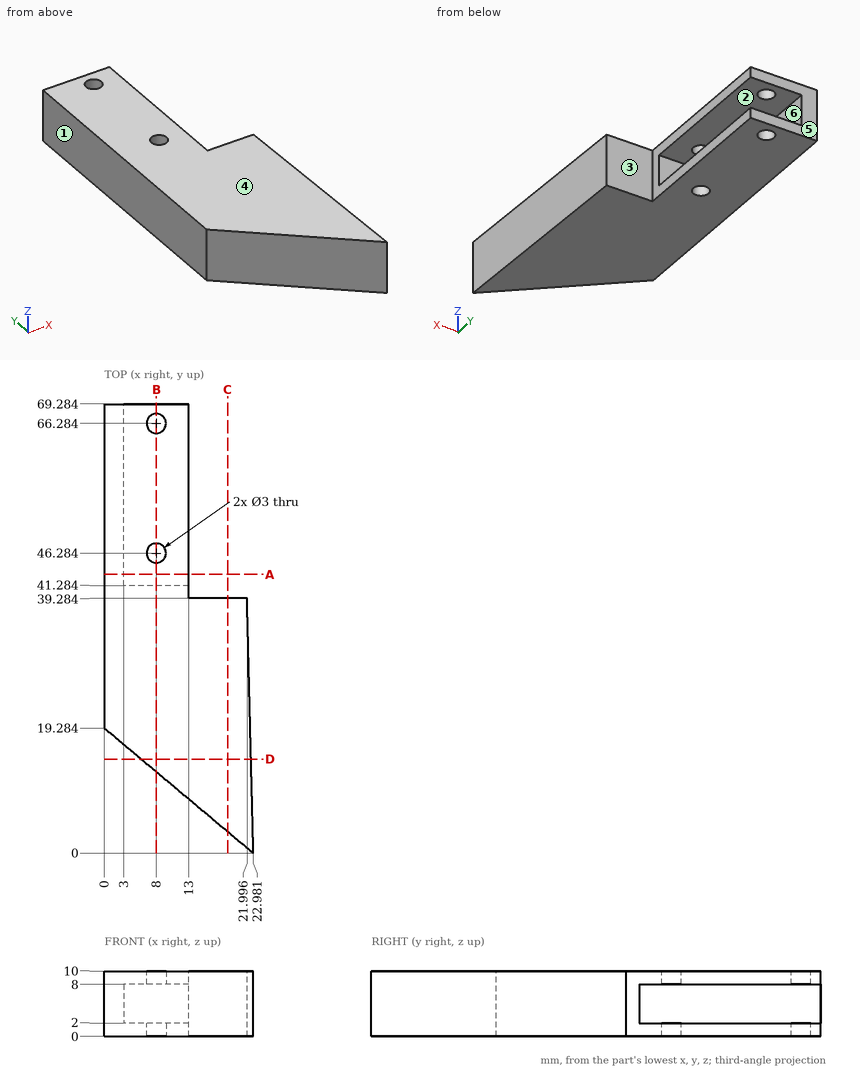
Verification items for this drawing (mm, ordinates from the low corner). A direction names the side the tool comes from. Give positions to 0.01 mm unless a question says otherwise; leave off trailing zeros. Loops run counter-clockwise (first coordinate to the right, second up) from the corner with the lowest first, then second, coordinate; pieces in that order, holes last. Notation, with made-up numbers: M 55,31.25 L 77,31.25 A25 cw 77,48.25 Z; hole C -7.75,48.25 d11. An arc over 180 degrees is marked long. Answer as CSV lines item,"result".
Item 1: Access from +Z, -Z, +X, -X, +Y, -Y to the whole of each face (thin tool, end or side, straight path). Record for the marked faces 1, 2 and 3.
Values:
face 1,"+Z, -Z, -X, +Y, -Y"
face 2,"+X, +Y"
face 3,"+Z, -Z, +X, +Y"
Item 2: Release check for a two-part mould opening along Z. For the marked faces 4, 5 and 6 record: pulls with the +Z half, pulls with the -Z half, needs draft (parallel to the pull), parting line crosses it, or undercut.
Values:
face 4,"pulls with the +Z half"
face 5,"needs draft"
face 6,"undercut"
Item 3: Cross-section at A-A on y = 43. Record the cut outline in (x, z).
Values:
outline,"M 0,0 L 13,0 L 13,2 L 3,2 L 3,8 L 13,8 L 13,10 L 0,10 Z"
Item 4: Depth check by flat-ended pin: P1, Ø2.5, axis at x = 8, y = 66.28, coming from the +Z side; P2, Ø6, axis at x = 16, y = 36, coming from the -Z side; P3, Ø1.8, axis at x = 10, z = 5, coming from the +Y side; P4, Ø3, axis at x = 11, z = 2, coming from the -Y side (1 decimal). Enter the tip coordinate at first touch or a pass-through.
Values:
P1,"passes through"
P2,"stops at z = 0"
P3,"stops at y = 41.28"
P4,"stops at y = 8.8"
Item 5: Cross-section at C-C on x = 19. Record the cut outline in (y, z).
Values:
outline,"M 3.34,0 L 39.28,0 L 39.28,10 L 3.34,10 Z"
Item 6: Cross-section at D-D on y = 14.5. Record the cut outline in (x, z).
Values:
outline,"M 5.7,0 L 22.62,0 L 22.62,10 L 5.7,10 Z"
Item 7: Cross-section at B-B on x = 8. Record the cut outline in (y, z), and give its area (3 significant figures).
Values:
outline,"M 12.57,0 L 44.78,0 L 44.78,2 L 41.28,2 L 41.28,8 L 44.78,8 L 44.78,10 L 12.57,10 Z; M 47.78,0 L 64.78,0 L 64.78,2 L 47.78,2 Z; M 47.78,8 L 64.78,8 L 64.78,10 L 47.78,10 Z; M 67.78,0 L 69.28,0 L 69.28,2 L 67.78,2 Z; M 67.78,8 L 69.28,8 L 69.28,10 L 67.78,10 Z"
area,"375 mm²"
Item 8: Material ranges on line 1 (Y direction, x = 8, z = 1.25) (1 decimal); line 2 (Z direction, x = 12.75, y = 53); line 3 (X direction, y = 49, z = 1.75), recorded low to high.
Values:
line 1,"y = 12.6 to 44.8, 47.8 to 64.8, 67.8 to 69.3"
line 2,"z = 0 to 2, 8 to 10"
line 3,"x = 0 to 13"
